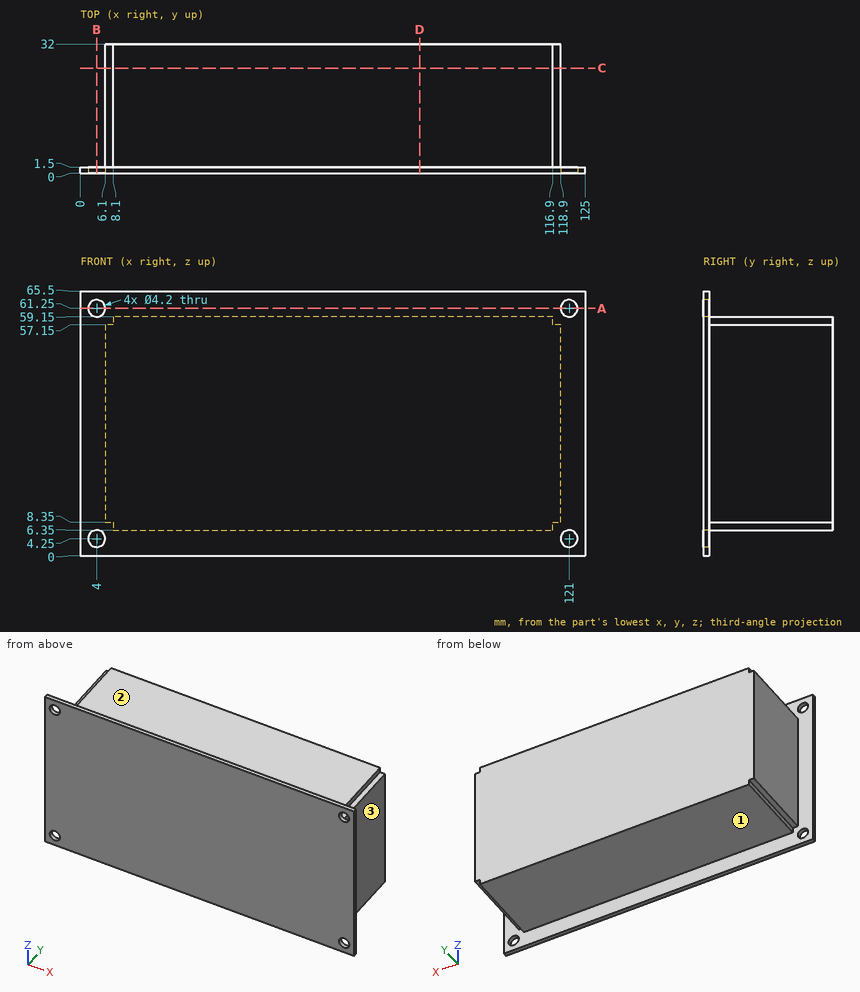
Here's the drawing with two shaded views (mm, measured from the low corner). I have some questions. A direction names the side the tool comes from. Coordinates: 2 decimals unless noted, no trailing zeros. Loops run counter-clockwise (first coordinate to the right, second up) from the corner with the lowest first, then second, coordinate; pieces in that order, holes last. Notation, with made-up numbers: (68.5, 13.25) -> (73.5, 13.25) arc R24 ccw to (73.5, 26.25) -> close; hole circle Ø5 at (65.5, 36). An arc over 180 degrees is marked (long way). Put each result on its own line as item: value. Start each with the question number.
Q1. If I drill on line 1 (Z direction, x = 121, y = 0.6); line 2 (X direction, y = 1.1, z = 61.25); line 3 (Z direction, x = 40, y = 22.5), over which ranges is the centre line in solid material (lowest first)? Write a range as [from, to].
Q2. I want a section at D-D (x = 84). Write out the boundary of the cut face in (y, z).
Q3. I want a section at A-A (z = 61.25). Write out the boundary of the cut face in (x, y).
Q4. I want a section at B-B (x = 4). Write out the boundary of the cut face in (y, z), plus the area to 4 significant figures.
Q5. For the marked faces 1, 2 and 3, which set-ups out of +Z, -Z, +X, -X, +Y, -Y let a thin tool reach every point of the face, with its end or its side?
Q6. I'm going to push flat-ended pins straight in: P1, Ø0.6, axis at x = 118.5, y = 18.5, coming from the +Z side; P2, Ø3, axis at y = 18, z = 56, coming from the +X side; P3, Ø1.6, axis at y = 18.5, z = 7.5, coming from the +X side. Where does each tip first touch, or does it pass through?
Q7. I want a section at C-C (y = 26). Write out the boundary of the cut face in (x, z), plus the area to 3 significant figures.
Taken from the geometry:
1. line 1: z = [0, 2.15], [6.35, 59.15], [63.35, 65.5]
1. line 2: x = [0, 1.9], [6.1, 118.9], [123.1, 125]
1. line 3: z = [6.35, 59.15]
2. outline: (0, 0) -> (1.5, 0) -> (1.5, 6.35) -> (32, 6.35) -> (32, 59.15) -> (1.5, 59.15) -> (1.5, 65.5) -> (0, 65.5) -> close
3. outline: (0, 0) -> (1.9, 0) -> (1.9, 1.5) -> (0, 1.5) -> close; (6.1, 0) -> (118.9, 0) -> (118.9, 1.5) -> (6.1, 1.5) -> close; (123.1, 0) -> (125, 0) -> (125, 1.5) -> (123.1, 1.5) -> close
4. outline: (0, 0) -> (1.5, 0) -> (1.5, 2.15) -> (0, 2.15) -> close; (0, 6.35) -> (1.5, 6.35) -> (1.5, 59.15) -> (0, 59.15) -> close; (0, 63.35) -> (1.5, 63.35) -> (1.5, 65.5) -> (0, 65.5) -> close
4. area: 85.65 mm2
5. face 1: -Z, +X, -X, +Y
5. face 2: +Z, +X, -X, +Y
5. face 3: +Z, -Z, +X, +Y
6. P1: stops at z = 57.15
6. P2: stops at x = 118.9
6. P3: stops at x = 116.9
7. outline: (6.1, 8.35) -> (8.1, 8.35) -> (8.1, 6.35) -> (116.9, 6.35) -> (116.9, 8.35) -> (118.9, 8.35) -> (118.9, 57.15) -> (116.9, 57.15) -> (116.9, 59.15) -> (8.1, 59.15) -> (8.1, 57.15) -> (6.1, 57.15) -> close
7. area: 5,940 mm2
